```python
from build123d import *

# Parameters (mm, degrees)
F1_DEPTH = 215.9
F2_R     = 2.54
F3_W     = 12.192
F3_H     = 0.254
F4_DEPTH = 215.901
F5_R     = 0.25399


# Not quite as in the source:
# - a fillet or chamfer is up to 0.001 mm smaller than in the source, because OpenCascade refuses the exact size


with BuildPart() as f1:
    # F0 (on Front) → F1 (new body)
    with BuildSketch(Plane.XZ):
        with BuildLine():
            Line((10.5184665114, -10.1497577667), (4.1684665114, -10.1497577667))
            Line((4.1684665114, -10.1497577667), (4.1684665114, -11.4197577667))
            ThreePointArc((4.1684665114, -11.4197577667), (4.8419857204, -11.6987385576), (5.1209665114, -12.3722577667))
            ThreePointArc((5.1209665114, -12.3722577667), (4.8419857204, -13.0457769758), (4.1684665114, -13.3247577667))
            Line((4.1684665114, -13.3247577667), (4.1684665114, -16.4997577667))
            Line((4.1684665114, -16.4997577667), (10.5184665114, -16.4997577667))
            Line((10.5184665114, -16.4997577667), (10.5184665114, -10.1497577667))
        make_face()
        with BuildLine():
            Line((16.8684665114, -10.1497577667), (10.5184665114, -10.1497577667))
            Line((10.5184665114, -10.1497577667), (10.5184665114, -16.4997577667))
            Line((10.5184665114, -16.4997577667), (16.8684665114, -16.4997577667))
            Line((16.8684665114, -16.4997577667), (16.8684665114, -13.3247577667))
            ThreePointArc((16.8684665114, -13.3247577667), (15.9159665114, -12.3722577667), (16.8684665114, -11.4197577667))
            Line((16.8684665114, -11.4197577667), (16.8684665114, -10.1497577667))
        make_face()
    extrude(amount=F1_DEPTH)

    # F2
    f2_edges = [f1.edges().sort_by_distance(p)[0] for p in [
        (16.868467, -107.95, -13.324758),
        (4.168467, -107.95, -13.324758),
    ]]
    fillet(f2_edges, radius=F2_R)

    # F3 (on face) → F4 (cut, through all)
    with BuildSketch(Plane.XZ.offset(215.9)):
        with Locations((10.5184665114, -10.2767577667)):
            Rectangle(F3_W, F3_H)
    extrude(amount=-F4_DEPTH, mode=Mode.SUBTRACT)

    # F5 (radius 0.254 in the source; OpenCascade refuses exactly that, so slightly less here)
    f5_edges = [f1.edges().sort_by_distance(p)[0] for p in [
        (4.422467, -107.95, -10.403758),
        (16.614467, -107.95, -10.403758),
        (16.868467, -107.95, -10.149758),
        (4.168467, -107.95, -10.149758),
    ]]
    fillet(f5_edges, radius=F5_R)


solid = f1.part
```
Work out the finished part from the listing and answer in its coordinate system (mm). Coordinates: 2 decimals unless noted, no trailing zeros. Write each loop counter-clockwise with the first axis right and the second up, starting at its lowest first coordinate (ties: lowest second). Pieces come first, ordered by that corner, then holes.
Q1. A cutting plane is placed at B-B, the plane x = 14. Give the vertices of the cut face in (y, z), then the cut area to 3 significant figures.
Q2. Each of these flat-tipped pins is pushed along its axis until it touches: pin 1 Ø1 at (y, z) = (-71, -13.5) entering from +X; pin 2 Ø2 at (x, y) = (14.5, -176) entering from +Z. Where does it stop, or does it pass through?
Q3. Determine the mould class of faces 1 (the face through (10, -106, -16.5)), 2 (the face through (10, -109, -10.404)) for opening direction X: released by +X, released by -X, zero draft, split by the parting line, or undercut.
Q4. Find the intervals of material crossed by line 1 (X direction, y = -40, z = -11.75); line 2 (X direction, y = -142.5, z = -13.75); line 3 (Z direction, x = 12.5, y = -139), in increasing order.
Findings below:
1. outline: (-215.9, -16.5) - (0, -16.5) - (0, -10.4) - (-215.9, -10.4) - close
1. area: 1,320 mm2
2. pin 1: stops at x = 16.75
2. pin 2: stops at z = -10.4
3. face 1: zero draft
3. face 2: undercut
4. line 1: x = 4.89 to 16.15
4. line 2: x = 4.38 to 16.65
4. line 3: z = -16.5 to -10.4
